Design review of the part built by this model. Coordinates are the model's own, in mm. Coordinates: 2 decimals unless noted, no trailing zeros. Loops run counter-clockwise (first coordinate to the right, second up) from the corner with the lowest first, then second, coordinate; pieces in that order, holes last. Notation, with made-up numbers: (10, 16.5) - (43, 16.5) arc R28 cw to (43, 44.5) - close; hole circle Ø3 at (-17.5, 87.5). An arc over 180 degrees is marked (long way). Answer in a Markdown table with one row per item. Add a question column.
(1) We need section B-B, the plane x = 24. Write out the cut boundary in (y, z), plus the area to 4 significant figures.
(2) We need section C-C, the plane z = 1. Give the number of separate pieces and of enclosed holes in the cut face, plus the area to 3 significant figures.
(3) To check wall thickness, follow L1, parallel to X at y = 212.5, z = 2.4 (3 decimals); L2, parallel to Y at x = 84, z = 2.85; L3, parallel to Y at x = 116.69, z = 2.05. State the ranges of each line that lie inside material, in increasing order. Write a range as [from, to].
(4) Clearance check with flat-ended pins moving along their axes: pin 1 (1.5 mm diameter, centred on x = 45, z = 2.5, fed in from +Y); pin 2 (1.5 mm diameter, centred on y = 292, z = 2, fed in from -X); pin 3 (1.5 mm diameter, centred on y = 192.5, z = 1.5, fed in from +X). State where each tip first meets the part, or that it passes through.
(5) We need section A-A, the plane y = 281.5. Write out the cut boundary in (x, z) (3 decimals), plus the area to 3 significant figures.
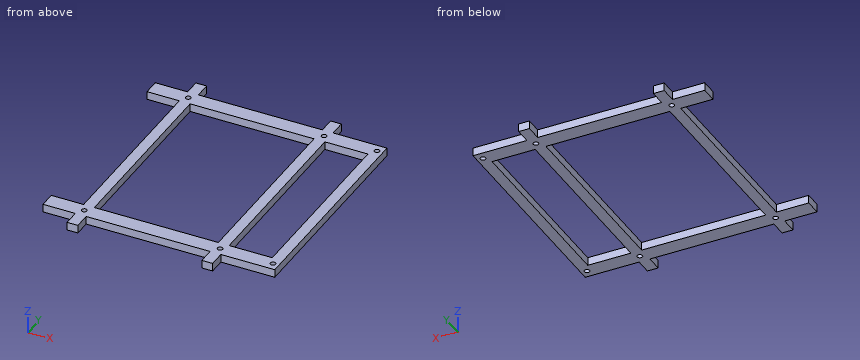
from build123d import *

# Parameters (mm, degrees)
F1_R     = 1.6
F1_W     = 76.668
F1_H     = 116
F1_W_2   = 26.667
F2_DEPTH = 5


with BuildPart() as f2:
    # F1 (on Top) → F2 (new body)
    with BuildSketch(Plane.XY):
        Polygon((-3.001, 187.310685), (3.666, 187.310685), (3.666, 197.310685), (80.334, 197.310685), (80.334, 187.310685), (87.001, 187.310685), (87.001, 197.310685), (113.668, 197.310685), (120.335, 197.310685), (120.335, 333.310685), (113.668, 333.310685), (87.001, 333.310685), (87.001, 343.310685), (80.334, 343.310685), (80.334, 333.310685), (3.666, 333.310685), (3.666, 343.310685), (-3.001, 343.310685), (-3.001, 333.310685), (-23.001, 333.310685), (-23.001, 323.310685), (-3.001, 323.310685), (-3.001, 207.310685), (-23.001, 207.310685), (-23.001, 197.310685), (-3.001, 197.310685), align=None)
        with Locations((0, 202.310685)):
            Circle(F1_R, mode=Mode.SUBTRACT)
        with Locations((42, 265.310685)):
            Rectangle(F1_W, F1_H, mode=Mode.SUBTRACT)
        with Locations((84, 202.310685)):
            Circle(F1_R, mode=Mode.SUBTRACT)
        with Locations((116.69, 202.310685)):
            Circle(F1_R, mode=Mode.SUBTRACT)
        with Locations((100.3345, 265.310685)):
            Rectangle(F1_W_2, F1_H, mode=Mode.SUBTRACT)
        with Locations((0, 328.310685)):
            Circle(F1_R, mode=Mode.SUBTRACT)
        with Locations((84, 328.310685)):
            Circle(F1_R, mode=Mode.SUBTRACT)
        with Locations((116.69, 328.310685)):
            Circle(F1_R, mode=Mode.SUBTRACT)
    extrude(amount=F2_DEPTH)


solid = f2.part
Responses:
| question | item | result |
|---|---|---|
| 1 | outline | (197.31, 0) - (207.31, 0) - (207.31, 5) - (197.31, 5) - close; (323.31, 0) - (333.31, 0) - (333.31, 5) - (323.31, 5) - close |
| 1 | area | 100.0 mm2 |
| 2 | separate pieces | 1 |
| 2 | enclosed holes | 8 |
| 2 | area | 5,410 mm2 |
| 3 | L1 | x = [-3.001, 3.666], [80.334, 87.001], [113.668, 120.335] |
| 3 | L2 | y = [187.31, 200.71], [203.91, 326.71], [329.91, 343.31] |
| 3 | L3 | y = [197.31, 200.71], [203.91, 326.71], [329.91, 333.31] |
| 4 | pin 1 | stops at y = 333.31 |
| 4 | pin 2 | stops at x = -3 |
| 4 | pin 3 | stops at x = 87 |
| 5 | outline | (-3.001, 0) - (3.666, 0) - (3.666, 5) - (-3.001, 5) - close; (80.334, 0) - (87.001, 0) - (87.001, 5) - (80.334, 5) - close; (113.668, 0) - (120.335, 0) - (120.335, 5) - (113.668, 5) - close |
| 5 | area | 100 mm2 |
